Here's how the part is built. I have some questions about the finished solid (model axes, mm). A direction names the side the tool comes from. Coordinates: 2 decimals unless noted, no trailing zeros. Write each loop counter-clockwise with the first axis right and the second up, starting at its lowest first coordinate (ties: lowest second). Pieces come first, ordered by that corner, then holes. Notation, with made-up numbers: M 47,68 L 101,68 A27 ccw 101,96 Z; hole C -34,87 d10. An arc over 180 degrees is marked long. Use a Markdown table: item, result.
```python
from build123d import *

# Parameters (mm, degrees)
SKETCH1_W                = 152.4
SKETCH1_H                = 101.6
BOSS_EXTRUDE1_DEPTH      = 6.35
CUT_EXTRUDE1_DEPTH       = 93.457395594
SKETCH3_W                = 152.4
SKETCH3_H                = 25.4
CUT_EXTRUDE2_DEPTH       = 93.457395594
G_0_261_DIAMETER_HOLE1_D = 6.6294
FILLET1_R                = 12.7


with BuildPart() as part:
    # Sketch1 → Boss-Extrude1 (new, symmetric)
    with BuildSketch(Plane.XY):
        Rectangle(SKETCH1_W, SKETCH1_H)
    extrude(amount=BOSS_EXTRUDE1_DEPTH, both=True)

    # Sketch2 → Cut-Extrude1 (cut, through all)
    with BuildSketch(Plane.XY.offset(6.35)):
        Polygon((0, 0), (50.8, 50.8), (-50.8, 50.8), align=None)
    extrude(amount=-CUT_EXTRUDE1_DEPTH, mode=Mode.SUBTRACT)

    # Sketch3 → Cut-Extrude2 (cut, through all)
    with BuildSketch(Plane.XY.offset(6.35)):
        with Locations((0, -38.1)):
            Rectangle(SKETCH3_W, SKETCH3_H)
    extrude(amount=-CUT_EXTRUDE2_DEPTH, mode=Mode.SUBTRACT)

    # G (0.261) Diameter Hole1 (through all)
    with Locations(Plane.XY.offset(6.35)):
        with Locations((-63.5, 38.1), (-63.5, -12.7), (63.5, -12.7), (63.5, 38.1)):
            Hole(G_0_261_DIAMETER_HOLE1_D / 2)

    # Fillet1
    fillet1_edges = [part.edges().sort_by_distance(p)[0] for p in [
        (0, 0, 0),
    ]]
    fillet(fillet1_edges, radius=FILLET1_R)


solid = part.part
```
1. Suppose I cut it at B-B on z = -4. Write out the boundary of the cut face in (x, y).
Answers follow:
| item | result |
|---|---|
| outline | M -76.2,-25.4 L 76.2,-25.4 L 76.2,50.8 L 50.8,50.8 L 8.98,8.98 A12.7 cw -8.98,8.98 L -50.8,50.8 L -76.2,50.8 Z; hole C -63.5,-12.7 d6.63; hole C -63.5,38.1 d6.63; hole C 63.5,-12.7 d6.63; hole C 63.5,38.1 d6.63 |
2. Suppose I cut it at A-A on y = -12.7. Write out the boundary of the cut face in (x, z), and give its area (3 significant figures).
Answers follow:
| item | result |
|---|---|
| outline | M -76.2,-6.35 L -66.81,-6.35 L -66.81,6.35 L -76.2,6.35 Z; M -60.19,-6.35 L 60.19,-6.35 L 60.19,6.35 L -60.19,6.35 Z; M 66.81,-6.35 L 76.2,-6.35 L 76.2,6.35 L 66.81,6.35 Z |
| area | 1,770 mm2 |
3. I need wall thicknesses on probe 1 along Y at (x, z) = (63.5, 2.75); probe 2 along Y at (x, z) = (65, 2.75); probe 3 along X at (y, z) = (7, -4.25). Which ranges of each line are inside material? Lowest first, please.
Answers follow:
| item | result |
|---|---|
| probe 1 | y = -25.4 to -16.01, -9.39 to 34.79, 41.41 to 50.8 |
| probe 2 | y = -25.4 to -15.66, -9.74 to 35.14, 41.06 to 50.8 |
| probe 3 | x = -76.2 to -6.42, 6.42 to 76.2 |
4. Suppose I cut it at D-D on y = 38.1. Write out the boundary of the cut face in (x, z).
Answers follow:
| item | result |
|---|---|
| outline | M -76.2,-6.35 L -66.81,-6.35 L -66.81,6.35 L -76.2,6.35 Z; M -60.19,-6.35 L -38.1,-6.35 L -38.1,6.35 L -60.19,6.35 Z; M 38.1,-6.35 L 60.19,-6.35 L 60.19,6.35 L 38.1,6.35 Z; M 66.81,-6.35 L 76.2,-6.35 L 76.2,6.35 L 66.81,6.35 Z |
5. Will these pins go through, and if not, where does the flat tip stop? pin 1 Ø2 at (x, z) = (45, 1.5) entering from +Y; pin 2 Ø2 at (x, z) = (24.5, -4) entering from +Y; pin 3 Ø1 at (x, z) = (-33, -0.5) entering from +Y.
Answers follow:
| item | result |
|---|---|
| pin 1 | stops at y = 46 |
| pin 2 | stops at y = 25.5 |
| pin 3 | stops at y = 33.5 |
6. Which directions (+Z, -Z, +X, -X, +Y, -Y) give clear straight access to the entire face, cutting with the end or side of a thin tool? Please do faces 4 (the face through (-30, 30, 0)), 5 (the face through (76.2, 12, 0)).
Answers follow:
| item | result |
|---|---|
| face 4 | +Z, -Z, +Y |
| face 5 | +Z, -Z, +X, +Y, -Y |
7. We'd pull the mould along Y, two halves only. Please class faces 1 (the face through (-65.03, 35.16, -0.09)), 2 (the face through (-76.2, 12, 0)), 3 (the face through (-0.14, 5.26, -0.09)): +Y half, -Y half, draft (parallel to the pull), parting line (faces both ways), or undercut.
Answers follow:
| item | result |
|---|---|
| face 1 | undercut |
| face 2 | draft |
| face 3 | +Y half |
8. Suppose I cut it at C-C on x = -63.5. Write out the boundary of the cut face in (y, z), and give its area (3 significant figures).
Answers follow:
| item | result |
|---|---|
| outline | M -25.4,-6.35 L -16.01,-6.35 L -16.01,6.35 L -25.4,6.35 Z; M -9.39,-6.35 L 34.79,-6.35 L 34.79,6.35 L -9.39,6.35 Z; M 41.41,-6.35 L 50.8,-6.35 L 50.8,6.35 L 41.41,6.35 Z |
| area | 799 mm2 |
